Build history of the part. All positions in model axes, mm. Coordinates: 2 decimals unless noted, no trailing zeros. Order: outer loops, then holes, each group sorted by start corner. A loop starts at its lowest first (then second) coordinate and runs counter-clockwise, first axis right, second up. Notation, with made-up numbers: M 45,8 L 74,8 A9 cw 74,13 Z; hole C 53.5,-24.5 d3. An arc over 180 degrees is marked long. Use a Markdown table: item, result. Add a question column.
Autodesk Inventor part; units mm, degrees
ref_plane "YZ Plane" through (0, 0, 0) normal (1, 0, 0) x (0, 1, 0)
ref_plane "XZ Plane" through (0, 0, 0) normal (0, 1, 0) x (-1, 0, 0)
ref_plane "XY Plane" through (0, 0, 0) normal (0, 0, 1) x (1, 0, 0)
sketch "Skizze1" plane through (0, 0, 0) normal (0, 0, 1) x (1, 0, 0)
  line L0 (-17.25, -3.75) -> (17.25, -3.75)
  line L1 (17.25, -3.75) -> (17.25, 3.75)
  line L2 (17.25, 3.75) -> (-17.25, 3.75)
  line L3 (-17.25, 3.75) -> (-17.25, -3.75)
  line L4 (-17.25, -3.75) -> (17.25, 3.75) construction
  line L5 (17.25, -3.75) -> (-17.25, 3.75) construction
  circle A0 centre (-12.5, 0) radius 1.7
  circle A1 centre (12.5, 0) radius 1.7
  line L6 (-17.25, 0) -> (17.25, 0) construction
  line L7 (0, -5.25) -> (0, 5.25) construction
  point P0 (0, 0)
  dimension "d0" = 7.5
  dimension "d1" = 34.5
  dimension "d2" = 3.4
  dimension "d3" = 25
extrude "Extrusion1" add sketch "Skizze1" along normal blind 3
properties part number "BMP280_Cableclamp"
(1) Slice it at C-C on z = 1.3. Give the cut face in (x, y).
(2) Slice it at A-A on x = 12.5. Give the cut face in (y, z), and give its area (3 significant figures).
(3) Drop a flat-ended pin along its axis: P1, Ø3, axis at x = 12.5, y = 0, coming from the +Z side. Give the stop position or say it passes through.
(4) Mould opens along Y. For faces 1 (the cylindrical face through (-10.93, 0.65, 1.48)), 2 (the flat face through (0, 0, 3)), 3 (the cylindrical face through (14.12, -0.51, 1.48)), 4 (the flat face through (0, 3.75, 1)) say: released by +Y, released by -Y, zero draft, split by the parting line, or undercut.
(5) Drill centre lines: line 1 along Y through (x, z) = (12.5, 2); line 2 along X through (y, z) = (0.5, 2); line 3 along X through (y, z) = (-1, 2.55). Where is each one in solid material? Low to high. Write a range as from..to.
(6) Slice it at B-B on y = -0.75. Give the cut face in (x, z).
Solutions:
| question | item | result |
|---|---|---|
| 1 | outline | M -17.25,-3.75 L 17.25,-3.75 L 17.25,3.75 L -17.25,3.75 Z; hole C -12.5,0 d3.4; hole C 12.5,0 d3.4 |
| 2 | outline | M -3.75,0 L -1.7,0 L -1.7,3 L -3.75,3 Z; M 1.7,0 L 3.75,0 L 3.75,3 L 1.7,3 Z |
| 2 | area | 12.3 mm² |
| 3 | P1 | through |
| 4 | face 1 | undercut |
| 4 | face 2 | zero draft |
| 4 | face 3 | undercut |
| 4 | face 4 | released by +Y |
| 5 | line 1 | -3.75..-1.7, 1.7..3.75 |
| 5 | line 2 | -17.25..-14.12, -10.88..10.88, 14.12..17.25 |
| 5 | line 3 | -17.25..-13.87, -11.13..11.13, 13.87..17.25 |
| 6 | outline | M -17.25,0 L -14.03,0 L -14.03,3 L -17.25,3 Z; M -10.97,0 L 10.97,0 L 10.97,3 L -10.97,3 Z; M 14.03,0 L 17.25,0 L 17.25,3 L 14.03,3 Z |
